```python
from build123d import *

# Parameters (mm, degrees)
SKETCH2_W               = 20
SKETCH2_H               = 3
CUT_EXTRUDE1_DEPTH      = 4
SKETCH3_W               = 20
SKETCH3_H               = 3
CUT_EXTRUDE2_DEPTH      = 4
SKETCH5_W               = 20
SKETCH5_H               = 0.8
CUT_EXTRUDE3_DEPTH      = 3.5
CUT_EXTRUDE3_DEPTH_BACK = 3.5


with BuildPart() as part:
    # Sketch1 → Revolve1 (revolve)
    with BuildSketch(Plane.XY):
        Polygon((0, 0), (0, 2.25), (0.25, 2.5), (19.5095, 2.5), (20, 2.0095), (20, 0), align=None)
    revolve(axis=Axis((20, 0, 0), (-1, 0, 0)))

    # Sketch2 → Cut-Extrude1 (cut)
    with BuildSketch(Plane(origin=(0, 0, 0), x_dir=(0, 0, -1), z_dir=(1, 0, 0))):
        with Locations((0, 3)):
            Rectangle(SKETCH2_W, SKETCH2_H)
    extrude(amount=CUT_EXTRUDE1_DEPTH, mode=Mode.SUBTRACT)

    # Sketch3 → Cut-Extrude2 (cut)
    with BuildSketch(Plane(origin=(0, 0, 0), x_dir=(0, 0, -1), z_dir=(1, 0, 0))):
        with Locations((0, -3)):
            Rectangle(SKETCH3_W, SKETCH3_H)
    extrude(amount=CUT_EXTRUDE2_DEPTH, mode=Mode.SUBTRACT)

    # Sketch4 → Cut-Revolve1 (revolve, cut)
    with BuildSketch(Plane.XY):
        Polygon((2, 1.5), (3.4, 1.5), (3, 1.1), (3, -1.1), (3.4, -1.5), (2, -1.5), align=None)
    revolve(axis=Axis((2, -1.5, 0), (0, 1, 0)), mode=Mode.SUBTRACT)

    # Sketch5 → Cut-Extrude3 (cut, two sides)
    with BuildSketch(Plane.XY) as cut_extrude3_sk:
        with Locations((10, 2.1)):
            Rectangle(SKETCH5_W, SKETCH5_H)
    extrude(amount=CUT_EXTRUDE3_DEPTH, mode=Mode.SUBTRACT)
    extrude(cut_extrude3_sk.sketch, amount=-CUT_EXTRUDE3_DEPTH_BACK, mode=Mode.SUBTRACT)


solid = part.part
```
The listing builds one solid part. Answer for the finished solid, in the listing's coordinates (mm). A direction names the side the tool comes from. Give positions to 0.01 mm unless a question says otherwise; leave off trailing zeros. Order: outer loops, then holes, each group sorted by start corner. A loop starts at its lowest first (then second) coordinate and runs counter-clockwise, first axis right, second up. Notation, with made-up numbers: (76, 19.25) - (125, 19.25) arc R13 cw to (125, 37.25) - close; hole circle Ø11 at (73, 42.25). An arc over 180 degrees is marked (long way). Answer in a Markdown table with one row per item. Add a question column.
Q1. Which of the six approach directions +Z, -Z, +X, -X, +Y, -Y give full straight-line access (tool end or side, diameter ignored) to faces 1 (the flat face through (1.1, -1.5, 1.4)), 2 (the conical face through (0.13, -0.02, 2.38)), 3 (the flat face through (0.6, 1.5, 0.9))?
Q2. The part is cut by section A-A (z = 0). Determine the outline of the cut face in (x, y).
Q3. Find the intervals of material crossed by line 1 along Z through (x, y) = (2, 0.15); line 2 along X through (y, z) = (0.3, 0); line 3 along X through (y, z) = (0.7, -0.4), in increasing order. Write a range as [from, to].
Q4. For a pull along Z with two mould halves and no side action, classify faces 4 (the conical face through (0.13, 0.02, -2.38)), 5 (the flat face through (4, -2, 0)), 6 (the cylindrical face through (1.2, 0, 0.6)) as released by +Z, released by -Z, zero draft, split by the parting line, or undercut.
Q5. The part is cut by section B-B (y = 0). Determine the outline of the cut face in (x, z), then the cut area to 3 significant figures.
Q6. The part is cut by section D-D (x = 12.25). Determine the outline of the cut face in (y, z).
Q7. Given P1, Ø3, axis at x = 2, z = 0, coming from the +Y side; P2, Ø1.6, axis at x = 2, z = 0, coming from the +Y side; P3, Ø0.8, axis at y = -2, z = 0.5, coming from the -X side, each flat-ended and moving along its own axis, determine where each tip first touches the part or whether it passes through.
Q8. The part is cut by section C-C (x = 2). Determine the outline of the cut face in (y, z).
Determined:
| question | item | result |
|---|---|---|
| 1 | face 1 | +Z, -Z, -X, -Y |
| 1 | face 2 | +Z, -X |
| 1 | face 3 | +Z, -Z, -X, +Y |
| 2 | outline | (0, -1.5) - (0.6, -1.5) - (1, -1.1) - (1, 1.1) - (0.6, 1.5) - (0, 1.5) - close; (3, -1.1) - (3.4, -1.5) - (4, -1.5) - (4, -2.5) - (19.51, -2.5) - (20, -2.01) - (20, 1.7) - (4, 1.7) - (4, 1.5) - (3.4, 1.5) - (3, 1.1) - close |
| 3 | line 1 | z = [-2.5, -1], [1, 2.5] |
| 3 | line 2 | x = [0, 1], [3, 20] |
| 3 | line 3 | x = [0, 1.08], [2.92, 20] |
| 4 | face 4 | released by -Z |
| 4 | face 5 | zero draft |
| 4 | face 6 | undercut |
| 5 | outline | (0, -2.25) - (0.25, -2.5) - (19.51, -2.5) - (20, -2.01) - (20, 2.01) - (19.51, 2.5) - (0.25, 2.5) - (0, 2.25) - close; hole circle Ø2 at (2, 0) |
| 5 | area | 96.6 mm² |
| 6 | outline | (1.7, -1.83) - (1.7, 1.83) arc R2.5 ccw (long way) to start |
| 7 | P1 | stops at y = 1.5 |
| 7 | P2 | passes through |
| 7 | P3 | stops at x = 4 |
| 8 | outline | (-1.5, -2) arc R2.5 ccw to (1.5, -2) - (1.5, -1.4) - (1.1, -1) - (-1.1, -1) - (-1.5, -1.4) - close; (-1.5, 1.4) - (-1.1, 1) - (1.1, 1) - (1.5, 1.4) - (1.5, 2) arc R2.5 ccw to (-1.5, 2) - close |
